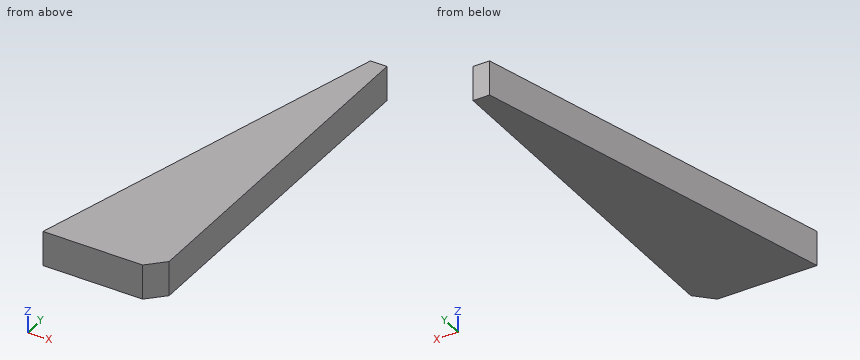
from build123d import *

# Parameters (mm, degrees)
BOSS_EXTRUDE1_DEPTH = 15


with BuildPart() as part:
    # Sketch1 → Boss-Extrude1 (new body)
    with BuildSketch(Plane.XY):
        Polygon((-50, 0), (-7.071067812, 0), (0, 7.071067812), (0, 160), (-7.128129211, 160), align=None)
    extrude(amount=-BOSS_EXTRUDE1_DEPTH)


solid = part.part
Check sheet for the modelled part. Datum: model origin and axes. Units: mm. Give positions to 0.01 mm unless a question says otherwise; leave off trailing zeros. Loops run counter-clockwise (first coordinate to the right, second up) from the corner with the lowest first, then second, coordinate; pieces in that order, holes last. Notation, with made-up numbers: M -22,17.25 L -2,17.25 A12 ccw -2,28.25 Z; hole C -35,65.25 d1. An arc over 180 degrees is marked long. Answer as a JSON object with one key per item and string values. Group by question number.
Q1. Cross-section at B-B on x = -13.5. Record the cut outline in (y, z), then the cut area to 3 significant figures.
Q2. Go/stop test with a flat-tipped pin: P1, Ø8, axis at y = 106.5, z = -9, coming from the -X side. Record where the tip stops, or that it passes through.
Q3. Cross-section at A-A on z = -4. Record the cut outline in (x, y).
Q4. Material ranges on line 1 along X through (y, z) = (76, -10); line 2 along X through (y, z) = (9.5, -5); line 3 along Y through (x, z) = (-6, -11), recorded low to high. Write a range as [from, to].
Q5. Cross-section at C-C on y = 133.5. Record the cut outline in (x, z), then the cut area to 3 significant figures.
Evaluation:
{
 "1": {"outline": "M 0,-15 L 136.22,-15 L 136.22,0 L 0,0 Z", "area": "2,040 mm2"},
 "2": {"P1": "stops at x = -22.54"},
 "3": {"outline": "M -50,0 L -7.07,0 L 0,7.07 L 0,160 L -7.13,160 Z"},
 "4": {"line 1": "x = [-29.64, 0]", "line 2": "x = [-47.45, 0]", "line 3": "y = [1.07, 160]"},
 "5": {"outline": "M -14.23,-15 L 0,-15 L 0,0 L -14.23,0 Z", "area": "213 mm2"}
}
